Answer from the drawing. Dimensions are ordinates in mm from the lowest x, y and z of the part. A direction names the side the tool comes from. Give positions to 0.01 mm unless a question says otherwise; leave off trailing zeros. Loops run counter-clockwise (first coordinate to the right, second up) from the corner with the lowest first, then second, coordinate; pieces in that order, holes last. Notation, with made-up numbers: (57, 59.25) -> (88, 59.25) arc R30 cw to (88, 91.25) -> close; hole circle Ø1 at (71, 58.25). An arc over 180 degrees is marked (long way). Return JSON: item names as keys, results as strings. Group by question number.
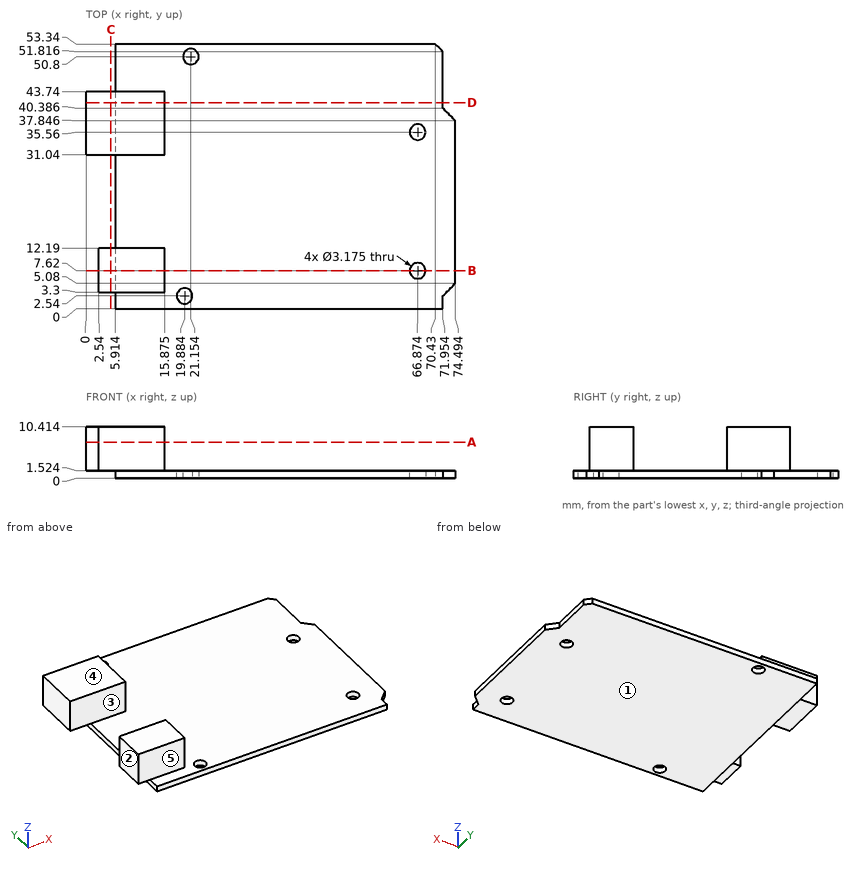
1. Straight lines are drawn through the part: line 1 (X direction, y = 4.5, z = 7.75) (1 decimal); line 2 (Z direction, x = 59, y = 42); line 3 (X direction, y = 41, z = 1). For each, find the intervals that lie inside material, in ascending order. Write a range as from..to.
2. Section B-B on y = 7.62 is taken. Determine the outline of the cut face in (x, z) (1 decimal), then the cut area to 3 significant figures.
3. Section D-D on y = 41.5 is taken. Determine the outline of the cut face in (x, z) (1 decimal).
4. Section C-C on x = 5 is taken. Determine the outline of the cut face in (y, z), then the cut area to 3 significant figures.
5. Determine the mould class of the marked faces 3, 4 and 5 for opening direction Y: pulls with the +Y half, pulls with the -Y half, needs draft (parallel to the pull), parting line crosses it, or undercut.
6. Which of the six approach directions +Z, -Z, +X, -X, +Y, -Y give full straight-line access (tool end or side, diameter ignored) to the marked faces 1 and 2?
7. Flat-ended cylindrical pins translate along their axes: pin 1 Ø10 at (x, y) = (64, 19) entering from -Z; pin 2 Ø4 at (x, y) = (66.87, 7.62) entering from +Z; pin 3 Ø2.5 at (x, z) = (6.5, 4.5) entering from +Y; pin 4 Ø3.5 at (x, y) = (4, 8.5) entering from -Z. Find the tip coordinate at first contact, or state that the pin passes through.
8. Section A-A on z = 7.25 is taken. Determine the outline of the cut face in (x, y) (1 decimal).
Completed:
{
 "1": {"line 1": "x = 2.5..15.9", "line 2": "z = 0..1.52", "line 3": "x = 5.91..71.95"},
 "2": {"outline": "(2.5, 1.5) -> (5.9, 1.5) -> (5.9, 0) -> (65.3, 0) -> (65.3, 1.5) -> (15.9, 1.5) -> (15.9, 10.4) -> (2.5, 10.4) -> close; (68.5, 0) -> (74.5, 0) -> (74.5, 1.5) -> (68.5, 1.5) -> close", "area": "218 mm²"},
 "3": {"outline": "(0, 1.5) -> (5.9, 1.5) -> (5.9, 0) -> (72, 0) -> (72, 1.5) -> (15.9, 1.5) -> (15.9, 10.4) -> (0, 10.4) -> close"},
 "4": {"outline": "(3.3, 1.52) -> (12.19, 1.52) -> (12.19, 10.41) -> (3.3, 10.41) -> close; (31.04, 1.52) -> (43.74, 1.52) -> (43.74, 10.41) -> (31.04, 10.41) -> close", "area": "192 mm²"},
 "5": {"face 3": "undercut", "face 4": "needs draft", "face 5": "pulls with the -Y half"},
 "6": {"face 1": "-Z, +X, -X, +Y, -Y", "face 2": "+Z, -Z, -X, -Y"},
 "7": {"pin 1": "stops at z = 0", "pin 2": "stops at z = 1.52", "pin 3": "stops at y = 43.74", "pin 4": "stops at z = 1.52"},
 "8": {"outline": "(0, 31) -> (15.9, 31) -> (15.9, 43.7) -> (0, 43.7) -> close; (2.5, 3.3) -> (15.9, 3.3) -> (15.9, 12.2) -> (2.5, 12.2) -> close"}
}
